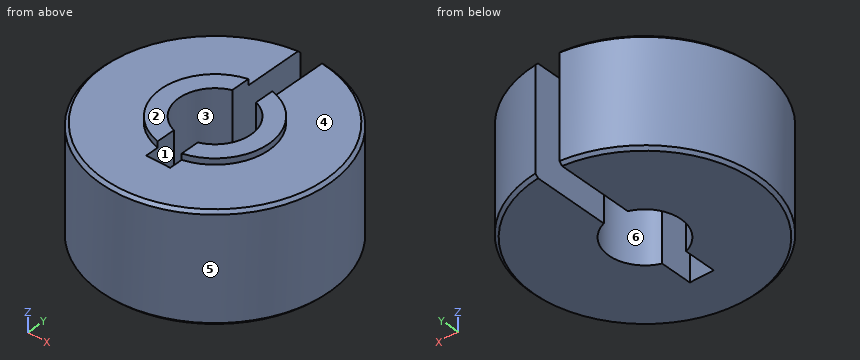
Autodesk Inventor part; units mm, degrees
ref_plane "YZ Plane" through (0, 0, 0) normal (1, 0, 0) x (0, 1, 0)
ref_plane "XZ Plane" through (0, 0, 0) normal (0, 1, 0) x (-1, 0, 0)
ref_plane "XY Plane" through (0, 0, 0) normal (0, 0, 1) x (1, 0, 0)
sketch "Base" plane through (0, 0, 0) normal (0, 0, 1) x (1, 0, 0)
  circle A0 centre (0, 0) radius 3
  circle A1 centre (0, 0) radius 9.5
  dimension "d0" = 6
  dimension "d1" = 19
extrude "Extrusion1" add sketch "Base" along normal blind 9
sketch "Sketch2" plane through (0, 0, 9) normal (0, 0, 1) x (1, 0, 0)
  circle A0 centre (0, 0) radius 4.5
  circle A1 centre (0, 0) radius 3
  dimension "d4" = 9
extrude "Extrusion2" add sketch "Sketch2" along normal blind 0.5
chamfer "Chamfer1" distance 0.25 angle 45 2 edges at (-9.5, 0, 9) (-9.5, 0, 0)
sketch "Sketch3" plane through (0, 0, 9) normal (0, 0, 1) x (1, 0, 0)
  line L0 (0, -5.5) -> (0, 9.5)
  circle A0 centre (0, 0) radius 9.5
  line L1 (-1, 9.5) -> (1, 9.5)
  line L2 (1, 9.5) -> (1, -5.5)
  line L3 (1, -5.5) -> (-1, -5.5)
  line L4 (-1, -5.5) -> (-1, 9.5)
  point P0 (-1, 9.4472)
  point P1 (1, 9.4472)
  dimension "d10" = 15
  dimension "d11" = 2
extrude "Extrusion3" cut sketch "Sketch3" against normal through all both and the other way through all contours L3 L4 A0 L0 | L0 A0 L2 L3
properties part number "ShoulderCollar"
Design review of the part built by this model. Coordinates are the model's own, in mm. Face numbers are marked on the shaded views. A direction names the side the tool comes from. Round coordinates to 2 decimals unless told otherwise and drop trailing zeros. Order: outer loops, then holes, each group sorted by start corner. A loop starts at its lowest first (then second) coordinate and runs counter-clockwise, first axis right, second up. Notation, with made-up numbers: M 48,5.25 L 94,5.25 A29 cw 94,30.25 Z; hole C 21,86 d5. An arc over 180 degrees is marked long. Answer as CSV lines item,"result". Start each with the question number.
1) For pin 1 Ø2 at (x, z) = (-3.5, 3.5) entering from +Y; pin 2 Ø5 at (y, z) = (4, 2) entering from -X; pin 3 Ø5.5 at (y, z) = (6.5, 2.5) entering from +X, all flat-tipped, find the tip position at first contact; note any pin that passes through.
2) Add section A-A (z = 9.25). Give the boundary of the cut face in (x, y).
3) Add section D-D (x = 0). Give the boundary of the cut face in (y, z).
4) Add section B-B (y = 0). Give the boundary of the cut face in (x, z), then the cut area to 3 significant figures.
5) Wall thickness on line 1 along Y through (x, z) = (-0.25, 1.5); line 2 along Z through (x, y) = (8.75, 0); line 3 along Y through (x, z) = (2, 4.75): over which ranges is each line inside the solid? List them lowest first. Write a range as [from, to].
6) Add section C-C (z = 5.5). Give the boundary of the cut face in (x, y), then the cut area to 3 significant figures.
7) Tool access review of the marked faces 1, 2 and 3: name each direction out of +Z, -Z, +X, -X, +Y, -Y from which nothing blocks a thin tool from reaching the whole face with its end or side.
8) The part is to be moulded in two halves that separate along Y. For the marked faces 4, 5 and 6, say which applies: +Y half, -Y half, draft (parallel to the pull), parting line (faces both ways), or undercut.
Resolved:
1,pin 1,"y = 9.17"
1,pin 2,"x = -9.38"
1,pin 3,"x = 8.73"
2,outline,"M -1,-4.39 L -1,-2.83 A3 cw -1,2.83 L -1,4.39 A4.5 ccw Z; M 1,-4.39 A4.5 ccw 1,4.39 L 1,2.83 A3 cw 1,-2.83 Z"
3,outline,"M -9.5,0.25 L -9.25,0 L -5.5,0 L -5.5,9 L -9.25,9 L -9.5,8.75 Z"
4,outline,"M -9.5,0.25 L -9.25,0 L -3,0 L -3,9.5 L -4.5,9.5 L -4.5,9 L -9.25,9 L -9.5,8.75 Z; M 3,0 L 9.25,0 L 9.5,0.25 L 9.5,8.75 L 9.25,9 L 4.5,9 L 4.5,9.5 L 3,9.5 Z"
4,area,"118 mm^2"
5,line 1,"[-9.5, -5.5]"
5,line 2,"[0, 9]"
5,line 3,"[-9.29, -2.24], [2.24, 9.29]"
6,outline,"M -1,-5.5 L -1,-2.83 A3 cw -1,2.83 L -1,9.45 A9.5 ccw long 1,9.45 L 1,2.83 A3 cw 1,-2.83 L 1,-5.5 Z"
6,area,"237 mm^2"
7,face 1,"+Z, -Z, +Y"
7,face 2,"+Z, +X, -X, +Y, -Y"
7,face 3,"+Z, -Z"
8,face 4,"draft"
8,face 5,"parting line"
8,face 6,"undercut"
